from build123d import *

# Parameters (mm, degrees)
EXTRUDE1_DEPTH     = 8.116924898
SKETCH2_W          = 56.161836645
SKETCH2_H          = 29.756220801
EXTRUDE2_DEPTH     = 3.825672251
SKETCH3_R          = 3.81
EXTRUDE3_DEPTH     = 22.721965672
SKETCH4_R          = 6.425
CUT_EXTRUDE1_DEPTH = 1.27
SKETCH6_R          = 1.638383055
EXTRUDE4_DEPTH     = 3.462479646
EXTRUDE5_DEPTH     = 24.392223233


with BuildPart() as part:
    # Sketch1 → Extrude1 (new, symmetric)
    with BuildSketch(Plane.XY):
        with BuildLine():
            Line((-7.138522943, -12.54381934), (-7.138522943, 0))
            ThreePointArc((-7.138522943, 0), (0, 7.138522943), (7.138522943, 0))
            Line((7.138522943, 0), (7.138522943, -12.54381934))
            Line((7.138522943, -12.54381934), (-7.138522943, -12.54381934))
        make_face()
    extrude(amount=EXTRUDE1_DEPTH, both=True)

    # Sketch2 → Extrude2 (cut, symmetric)
    with BuildSketch(Plane.XY):
        with Locations((-1.286243087, 9.527651968)):
            Rectangle(SKETCH2_W, SKETCH2_H)
    extrude(amount=EXTRUDE2_DEPTH, both=True, mode=Mode.SUBTRACT)

    # Sketch3 → Extrude3 (cut, through all)
    with BuildSketch(Plane.XY.offset(8.116924898)):
        Circle(SKETCH3_R)
    extrude(amount=-EXTRUDE3_DEPTH, mode=Mode.SUBTRACT)

    # Sketch4 → Cut-Extrude1 (cut)
    with BuildSketch(Plane.XZ.offset(12.54381934)):
        Circle(SKETCH4_R)
    extrude(amount=-CUT_EXTRUDE1_DEPTH, mode=Mode.SUBTRACT)

    # Sketch6 → Extrude4 (add, symmetric)
    with BuildSketch(Plane.XY):
        with BuildLine():
            Line((7.138522943, -12.54381934), (7.138522943, -5.350458433))
            Line((7.138522943, -5.350458433), (12.396008331, -5.350458433))
            ThreePointArc((12.396008331, -5.350458433), (15.992688785, -8.947138887), (12.396008331, -12.54381934))
            Line((12.396008331, -12.54381934), (7.138522943, -12.54381934))
        make_face()
        with Locations((12.396008331, -8.947138887)):
            Circle(SKETCH6_R, mode=Mode.SUBTRACT)
    extrude4 = extrude(amount=EXTRUDE4_DEPTH, both=True)

    # Mirror1: Extrude4 across plane
    add(extrude4.mirror(Plane(origin=(0, 0, 0), x_dir=(0, 0, 1), z_dir=(1, 0, 0))))

    # Sketch7 → Extrude5 (cut, through all)
    with BuildSketch(Plane.XY.offset(3.462479646)):
        with BuildLine():
            Line((7.138522943, -12.54381934), (12.396008331, -12.54381934))
            ThreePointArc((12.396008331, -12.54381934), (15.992688785, -8.947138887), (12.396008331, -5.350458433))
            Line((12.396008331, -5.350458433), (7.138522943, -5.350458433))
            Line((7.138522943, -5.350458433), (7.138522943, -12.54381934))
        make_face()
    extrude(amount=-EXTRUDE5_DEPTH, mode=Mode.SUBTRACT)


solid = part.part
Can you work these out from the model? Positions are in its coordinate system, mm. A direction names the side the tool comes from. Coordinates: 2 decimals unless noted, no trailing zeros. Loops run counter-clockwise (first coordinate to the right, second up) from the corner with the lowest first, then second, coordinate; pieces in that order, holes last. Notation, with made-up numbers: M 15,78 L 56,78 A21 cw 56,83 Z; hole C 33.25,51 d6. An arc over 180 degrees is marked long. Return JSON: item names as keys, results as strings. Group by question number.
Item 1: Imagine slicing it at A-A (x = 0). Please give me the cut outline in (y, z) (3 decimals).
Item 2: I'm going to push flat-ended pins straight in: pin 1 Ø6 at (y, z) = (2, 1) entering from +X; pin 2 Ø4 at (x, z) = (3, -1.5) entering from -Y; pin 3 Ø2 at (x, y) = (-11.5, -8.5) entering from -Z. Where does each tip first touch, or does it pass through?
Item 3: Imagine slicing it at D-D (y = 2). Please give me the cut outline in (x, z), and give its area (3 significant figures).
Item 4: Imagine slicing it at C-C (z = -7). Please give me the cut outline in (x, y), and give its area (3 significant figures).
Item 5: Thinking about a two-plate mould opening in Z: for faces 1 (the flat face through (-10.6, -8.9, 3.462)), 2 (the flat face through (-2, 4, 3.826)), 3 (the flat face through (7.139, -8, 0)), which applies, released by +Z, released by -Z, zero draft, split by the parting line, or undercut?
Item 6: Imagine slicing it at B-B (y = 4.25). Please give me the cut outline in (x, z), and give its area (4 significant figures).
Item 7: If I drill on L1, parallel to Y at x = 0, z = -5.9; L2, parallel to Z at x = -6.5, y = -2.75; L3, parallel to Z at x = 0, y = -11.8 (3 decimals), over which ranges is the centre line in solid material (lowest first)? Write a range as from..to.
Item 8: On a 3-axis mill with a long thin cutter (end or side, diameter ignored), from which of +Z, -Z, +X, -X, +Y, -Y can I reach the whole of each face in a straight line? I mean faces 4 (the flat face through (0, -11.274, 0)), 5 (the flat face through (-7.139, -6, 6)), 6 (the flat face through (-2, 4, -3.826)). Say none if no direction works.
Verdict:
{
 "1": {"outline": "M -12.544,-8.117 L -3.81,-8.117 L -3.81,-3.826 L -5.35,-3.826 L -5.35,3.826 L -3.81,3.826 L -3.81,8.117 L -12.544,8.117 L -12.544,6.425 L -11.274,6.425 L -11.274,-6.425 L -12.544,-6.425 Z; M 3.81,-8.117 L 7.139,-8.117 L 7.139,-3.826 L 3.81,-3.826 Z; M 3.81,3.826 L 7.139,3.826 L 7.139,8.117 L 3.81,8.117 Z"},
 "2": {"pin 1": "stops at x = 7.07", "pin 2": "stops at y = -11.27", "pin 3": "stops at z = -3.46"},
 "3": {"outline": "M -6.85,-8.12 L -3.24,-8.12 L -3.24,-3.83 L -6.85,-3.83 Z; M -6.85,3.83 L -3.24,3.83 L -3.24,8.12 L -6.85,8.12 Z; M 3.24,-8.12 L 6.85,-8.12 L 6.85,-3.83 L 3.24,-3.83 Z; M 3.24,3.83 L 6.85,3.83 L 6.85,8.12 L 3.24,8.12 Z", "area": "62.0 mm^2"},
 "4": {"outline": "M -7.14,-12.54 L 7.14,-12.54 L 7.14,0 A7.14 ccw -7.14,0 Z; hole C 0,0 d7.62", "area": "214 mm^2"},
 "5": {"face 1": "released by +Z", "face 2": "undercut", "face 3": "zero draft"},
 "6": {"outline": "M -5.74,-8.12 L 5.74,-8.12 L 5.74,-3.83 L -5.74,-3.83 Z; M -5.74,3.83 L 5.74,3.83 L 5.74,8.12 L -5.74,8.12 Z", "area": "98.45 mm^2"},
 "7": {"L1": "y = -11.27..-3.81, 3.81..7.14", "L2": "z = -8.12..-3.83, 3.83..8.12", "L3": "z = -8.117..-6.425, 6.425..8.117"},
 "8": {"face 4": "-Y", "face 5": "+Z, -X, +Y, -Y", "face 6": "+X, -X, +Y"}
}
